from build123d import *

# Parameters (mm, degrees)
SKETCH1_R           = 11
BOSS_EXTRUDE1_DEPTH = 49
SKETCH2_R           = 1
CUT_EXTRUDE1_DEPTH  = 3
SKETCH3_R           = 3
BOSS_EXTRUDE2_DEPTH = 6


with BuildPart() as part:
    # Sketch1 → Boss-Extrude1 (new body)
    with BuildSketch(Plane.XY):
        Circle(SKETCH1_R)
    extrude(amount=BOSS_EXTRUDE1_DEPTH)

    # Sketch2 → Cut-Extrude1 (cut)
    with BuildSketch(Plane.XY.offset(49)):
        with Locations((6.875, 0)):
            Circle(SKETCH2_R)
        with Locations((0, -6.875)):
            Circle(SKETCH2_R)
        with Locations((-6.875, 0)):
            Circle(SKETCH2_R)
        with Locations((0, 6.875)):
            Circle(SKETCH2_R)
    extrude(amount=-CUT_EXTRUDE1_DEPTH, mode=Mode.SUBTRACT)

    # Sketch3 → Boss-Extrude2 (add)
    with BuildSketch(Plane.XY.offset(49)):
        Circle(SKETCH3_R)
    extrude(amount=BOSS_EXTRUDE2_DEPTH)


solid = part.part
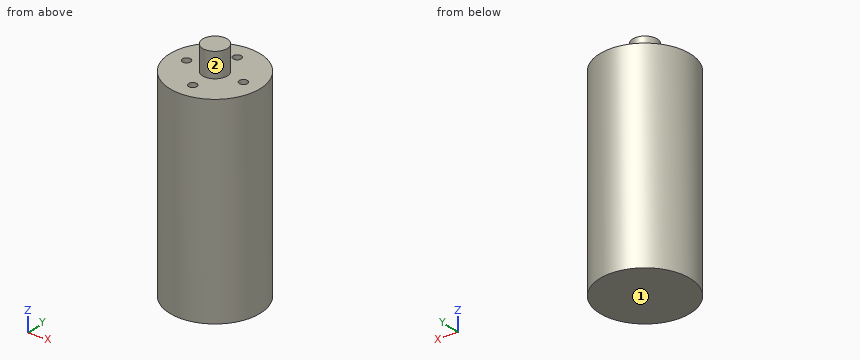
The model under review builds one solid part; all positions refer to its coordinate system, in mm. Face numbers are marked on the shaded views. A direction names the side the tool comes from. Round coordinates to 2 decimals unless told otherwise and drop trailing zeros. Write each loop counter-clockwise with the first axis right and the second up, starting at its lowest first coordinate (ties: lowest second). Pieces come first, ordered by that corner, then holes. Notation, with made-up numbers: (79, 43) - (88, 43) arc R15 cw to (88, 61) - close; hole circle Ø7 at (53, -2). An arc over 180 degrees is marked (long way). One line per item, written item: value. Start each with the question number.
1. Consider section C-C on z = 11.5. Write out the cut boundary in (x, y).
2. Clearance check with flat-ended pins moving along their axes: P1, Ø1, axis at x = -0.5, y = -6.5, coming from the +Z side; P2, Ø1.2, axis at x = 0, y = -6.875, coming from the +Z side; P3, Ø4, axis at x = -8, y = 2, coming from the -Z side; P4, Ø1.5, axis at y = 7, z = 14.5, coming from the +X side. State where each tip first meets the part, or that it passes through.
3. Machinability: for the marked faces 1 and 2, which of the approach directions +Z, -Z, +X, -X, +Y, -Y give a long, thin tool a straight path to every point of the face, cutting with its end or side? Answer none if there is none.
4. Consider section D-D on x = -9.5. Write out the cut boundary in (y, z).
5. Consider section A-A on x = 0. Write out the cut boundary in (y, z) (3 decimals), and give its area (3 significant figures).
6. To check wall thickness, follow L1, parallel to Y at x = 0, z = 47.8 (3 decimals); L2, parallel to Z at x = 1.5, y = -7.25; L3, parallel to Z at x = -6.75, y = 0.75. State the ranges of each line that lie inside material, in increasing order. Write a range as from..to.
Checks:
1. outline: circle Ø22 at (0, 0)
2. P1: stops at z = 49
2. P2: stops at z = 46
2. P3: stops at z = 0
2. P4: stops at x = 9.05
3. face 1: -Z, +X, -X, +Y, -Y
3. face 2: +Z
4. outline: (-5.55, 0) - (5.55, 0) - (5.55, 49) - (-5.55, 49) - close
5. outline: (-11, 0) - (11, 0) - (11, 49) - (7.875, 49) - (7.875, 46) - (5.875, 46) - (5.875, 49) - (3, 49) - (3, 55) - (-3, 55) - (-3, 49) - (-5.875, 49) - (-5.875, 46) - (-7.875, 46) - (-7.875, 49) - (-11, 49) - close
5. area: 1,100 mm^2
6. L1: y = -11..-7.875, -5.875..5.875, 7.875..11
6. L2: z = 0..49
6. L3: z = 0..46
